The drawing under review shows one solid part. Ordinate dimensions are in mm from its lowest x, y, z. A direction names the side the tool comes from. Give positions to 0.01 mm unless a question says otherwise; leave off trailing zeros. Loops run counter-clockwise (first coordinate to the right, second up) from the corner with the lowest first, then second, coordinate; pieces in that order, holes last. Notation, with made-up numbers: M 72.25,40.5 L 129.25,40.5 A20 ccw 129.25,48.5 Z; hole C 47.25,75 d3. An arc over 180 degrees is marked long. Write item = value, one per line. Start each with the question number.
1. For pin 1 (1.5 mm diameter, centred on x = 2.5, y = 3.5, fed in from -Z); pin 2 (1 mm diameter, centred on x = 7.5, y = 2.5, fed in from +Z), all flat-tipped, find the tip position at first contact; note any pin that passes through.
2. We need section A-A on z = 2. Give the boundary of the cut face in (x, y), then the cut area to 3 significant figures.
3. We need section C-C on x = 7. Give the boundary of the cut face in (y, z).
4. For the marked faces 1 and 2, list the 3-axis set-ups (+Z, -Z, +X, -X, +Y, -Y) from which the entire face can be reached by the end or side of a thin tool; tool diameter is ignored.
5. Wall thickness on line 1 along Y through (x, z) = (7.5, 1.5); line 2 along X through (y, z) = (3.2, 1.3); line 3 along Y through (x, z) = (9.75, 2.9): over which ranges is each line inside the solid? List them lowest first. Write a range as from..to.
6. We need section B-B on x = 1. Give the boundary of the cut face in (y, z).
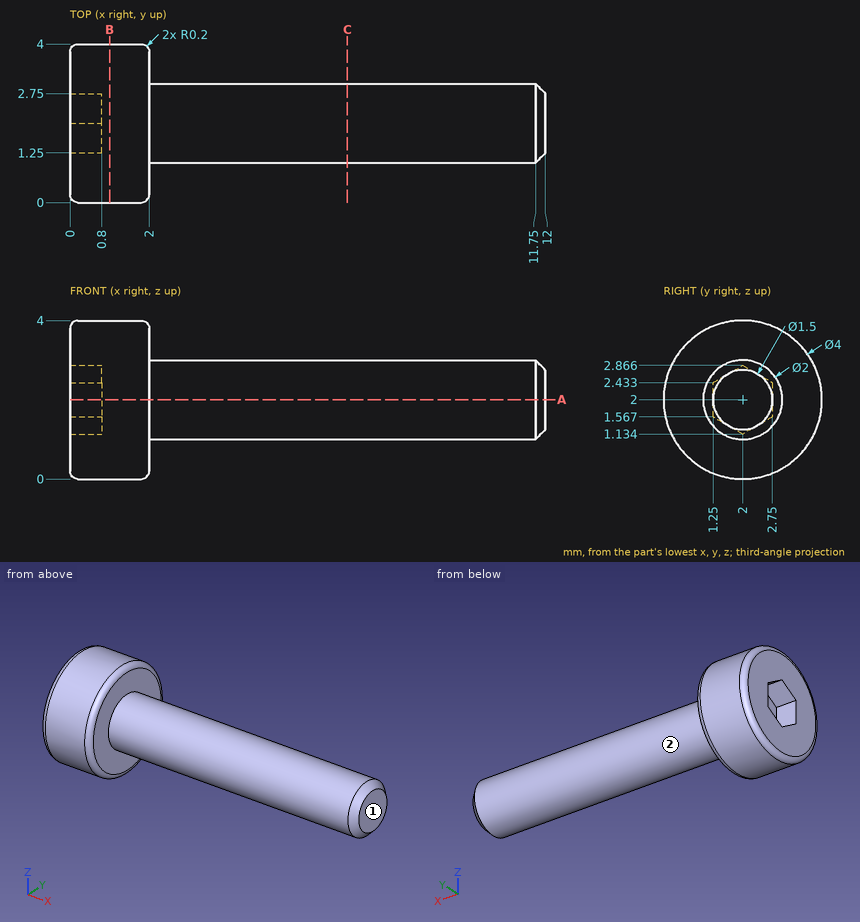
Final values:
q1.pin_1 = 0.33
q1.pin_2 = 3
q2.outline = M 0,0.2 A0.2 ccw 0.2,0 L 1.8,0 A0.2 ccw 2,0.2 L 2,1 L 11.75,1 L 12,1.25 L 12,2.75 L 11.75,3 L 2,3 L 2,3.8 A0.2 ccw 1.8,4 L 0.2,4 A0.2 ccw 0,3.8 L 0,2.75 L 0.8,2.75 L 0.8,1.25 L 0,1.25 Z
q2.area = 26.7 mm²
q3.outline = C 2,2 d2
q4.face_1 = +Z, -Z, +X, +Y, -Y
q4.face_2 = +X
q5.line_1 = 1.13..2.87
q5.line_2 = 0..2
q5.line_3 = 1.56..2.44
q6.outline = C 2,2 d4
